from build123d import *

# Parameters (mm, degrees)
F1_DEPTH = 25.4
F2_DEPTH = 12.7
F3_W     = 14.980048
F3_H     = 12.7
F4_DEPTH = 6.35


with BuildPart() as f1:
    # F0 (on Right) → F1 (new body)
    with BuildSketch(Plane.YZ):
        Polygon((-25.4, 0), (0, 0), (0, 31.75), (-12.7, 31.75), (-12.7, 12.7), (-25.4, 12.7), align=None)
    extrude(amount=F1_DEPTH)

    # F1_face (on face) → F2 (join)
    with BuildSketch(Plane(origin=(25.4, -9.978571, 13.153571), x_dir=(0, 1, 0), z_dir=(1, 0, 0))):
        Polygon((-15.421429, -13.153571), (9.978571, -13.153571), (9.978571, 18.596429), (-2.721429, 18.596429), (-2.721429, -0.453571), (-15.421429, -0.453571), align=None)
    extrude(amount=F2_DEPTH)

    # F3 (on face) → F4 (cut)
    with BuildSketch(Plane.XY.offset(31.75)):
        with Locations((17.623421, -6.35)):
            Rectangle(F3_W, F3_H)
    extrude(amount=-F4_DEPTH, mode=Mode.SUBTRACT)


solid = f1.part
Can you work these out from the model? Positions are in its coordinate system, mm. A direction names the side the tool comes from. Coordinates: 2 decimals unless noted, no trailing zeros. Write each loop counter-clockwise with the first axis right and the second up, starting at its lowest first coordinate (ties: lowest second). Pieces come first, ordered by that corner, then holes. Notation, with made-up numbers: (84, -6) - (102, -6) arc R6 cw to (102, 1) - close; hole circle Ø8 at (-18, 53.25). An arc over 180 degrees is marked (long way). Return JSON: item names as keys, results as strings. Group by question number.
Item 1: We'd pull the mould along X, two halves only. Please class faces 1 (the face through (19, -13, 0)), 2 (the face through (0, -10, 13)), 3 (the face through (10.133, -6, 29)), 4 (the face through (18, -6, 25.4)): pulls with the +X half, pulls with the -X half, needs draft (parallel to the pull), parting line crosses it, or undercut.
Item 2: I'm going to push flat-ended pins straight in: pin 1 Ø12 at (x, z) = (31, 20) entering from -Y; pin 2 Ø10 at (x, y) = (16.5, -4) entering from +Z; pin 3 Ø1.5 at (x, y) = (7, -17) entering from +Z. Where does each tip first touch, or does it pass through?
Item 3: If we section it at A-A (x = 32): Write out the boundary of the cut face in (y, z).
Item 4: Which directions (+Z, -Z, +X, -X, +Y, -Y) give clear straight access to the entire face, cutting with the end or side of a thin tool? Please do faces 5 (the face through (19, -12.7, 20)), 6 (the face through (5, -6, 31.75)), 7 (the face through (25.113, -6, 29)).
Item 5: If we section it at C-C (z = 14.5): Write out the boundary of the cut face in (x, y).
Item 6: If we section it at B-B (y = -5.25): Write out the boundary of the cut face in (x, z).
Item 7: If we section it at D-D (x = 15.5): Write out the boundary of the cut face in (y, z), then the cut area to 3 significant figures.
Item 8: Please list where these lines run through material, in increasing order: probe 1 along Z at (x, y) = (13, -9.25); probe 2 along Y at (x, z) = (5.5, 18); probe 3 along Z at (x, y) = (25.5, -19.5).
Return value:
{
 "1": {"face 1": "needs draft", "face 2": "pulls with the -X half", "face 3": "undercut", "face 4": "undercut"},
 "2": {"pin 1": "stops at y = -12.7", "pin 2": "stops at z = 25.4", "pin 3": "stops at z = 12.7"},
 "3": {"outline": "(-25.4, 0) - (0, 0) - (0, 31.75) - (-12.7, 31.75) - (-12.7, 12.7) - (-25.4, 12.7) - close"},
 "4": {"face 5": "+Z, +X, -X, -Y", "face 6": "+Z, +X, -X, +Y, -Y", "face 7": "+Z, +Y, -Y"},
 "5": {"outline": "(0, -12.7) - (38.1, -12.7) - (38.1, 0) - (0, 0) - close"},
 "6": {"outline": "(0, 0) - (38.1, 0) - (38.1, 31.75) - (25.11, 31.75) - (25.11, 25.4) - (10.13, 25.4) - (10.13, 31.75) - (0, 31.75) - close"},
 "7": {"outline": "(-25.4, 0) - (0, 0) - (0, 25.4) - (-12.7, 25.4) - (-12.7, 12.7) - (-25.4, 12.7) - close", "area": "484 mm^2"},
 "8": {"probe 1": "z = 0 to 25.4", "probe 2": "y = -12.7 to 0", "probe 3": "z = 0 to 12.7"}
}
